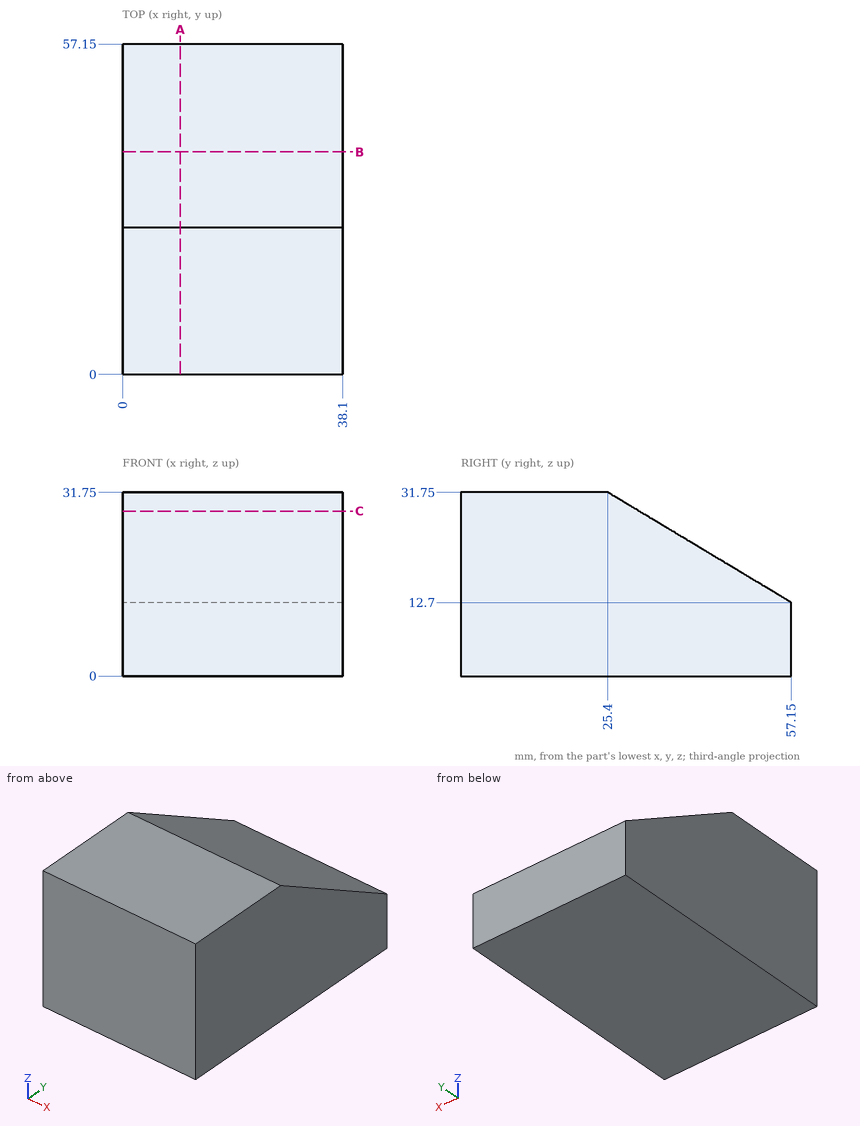
Source: three-view drawing plus pictorial views. Frame: mm from the lowest corner of the part. Coordinates: 2 decimals unless noted, no trailing zeros. Order: outer loops, then holes, each group sorted by start corner. A loop starts at its lowest first (then second) coordinate and runs counter-clockwise, first axis right, second up. Notation, with made-up numbers: M 74.25,51.5 L 128.25,51.5 A8 cw 128.25,57.5 Z; hole C -23.75,61.5 d4. An arc over 180 degrees is marked long. Answer in a Markdown table with one row per item.
(1) Material intervals for line 1 (Y direction, x = 33, z = 29.5); line 2 (Y direction, x = 4, z = 16); line 3 (Z direction, x = 32, y = 39.5), sorted ascending. Write a range as [from, to].
Numbers:
| item | result |
|---|---|
| line 1 | y = [0, 29.15] |
| line 2 | y = [0, 51.65] |
| line 3 | z = [0, 23.29] |
(2) Section query A-A, the plane x = 10. Output: boundary loops of the cut face in (y, z).
Numbers:
| item | result |
|---|---|
| outline | M 0,0 L 57.15,0 L 57.15,12.7 L 25.4,31.75 L 0,31.75 Z |
(3) Contact query for flat-ended pins moving along their axis: pin 1 Ø5 at (x, y) = (19, 45.5) entering from +Z; pin 2 Ø3 at (x, z) = (7, 26.5) entering from +Y; pin 3 Ø1.5 at (x, y) = (20.5, 44.5) entering from +Z. Output: stop coordinate, or through.
Numbers:
| item | result |
|---|---|
| pin 1 | stops at z = 21.19 |
| pin 2 | stops at y = 36.65 |
| pin 3 | stops at z = 20.74 |
(4) Section query C-C, the plane z = 28.5. Output: boundary loops of the cut face in (x, y), plus the area to 3 significant figures.
Numbers:
| item | result |
|---|---|
| outline | M 0,0 L 38.1,0 L 38.1,30.82 L 0,30.82 Z |
| area | 1,170 mm^2 |
(5) Section query B-B, the plane y = 38.5. Output: boundary loops of the cut face in (x, z).
Numbers:
| item | result |
|---|---|
| outline | M 0,0 L 38.1,0 L 38.1,23.89 L 0,23.89 Z |
